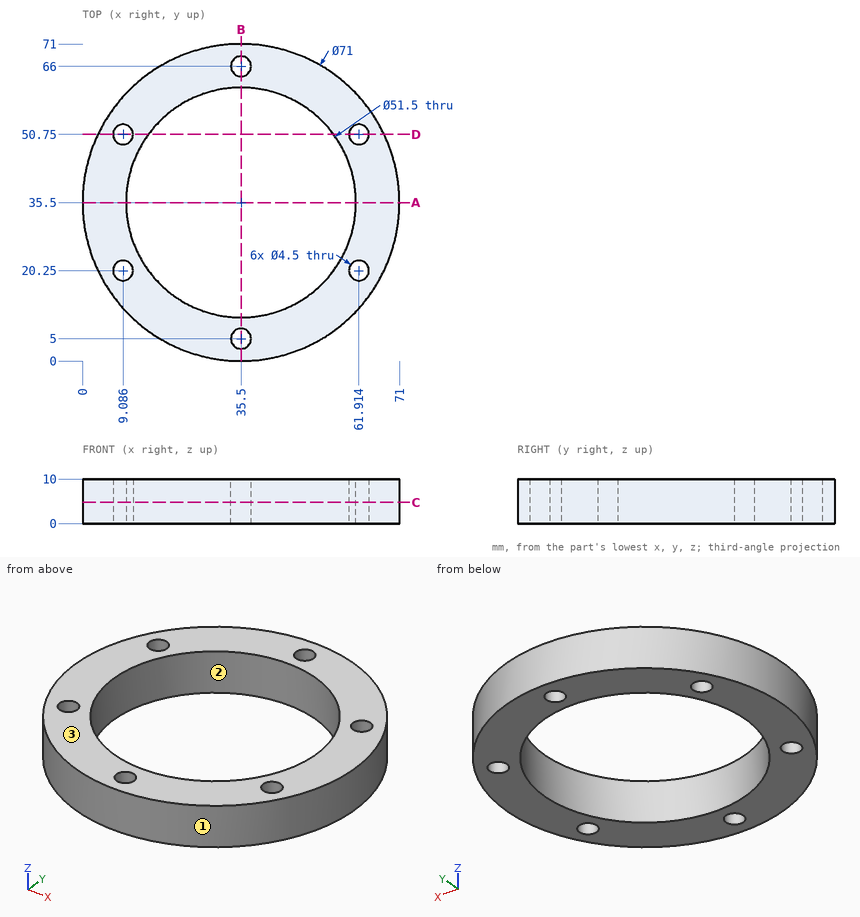
Study the drawing (mm; zero at the part's minimum x, y, z) and answer. Coordinates: 2 decimals unless noted, no trailing zeros. Write each loop counter-clockwise with the first axis right and the second up, starting at its lowest first coordinate (ties: lowest second). Pieces come first, ordered by that corner, then holes. Notation, with made-up numbers: M 51,2 L 84,2 A27 cw 84,41 Z; hole C 28,-39 d4. An arc over 180 degrees is marked long. Write each question's results on one line, items separated by ' | '.
Item 1: The part is cut by section C-C on z = 4.75. Determine the outline of the cut face in (x, y).
Answer below:
outline: C 35.5,35.5 d71; hole C 9.09,20.25 d4.5; hole C 9.09,50.75 d4.5; hole C 35.5,35.5 d51.5; hole C 35.5,5 d4.5; hole C 35.5,66 d4.5; hole C 61.91,20.25 d4.5; hole C 61.91,50.75 d4.5
Item 2: Given P1, Ø6, axis at x = 61.91, y = 20.25, coming from the -Z side; P2, Ø1.5, axis at x = 41.5, z = 4.5, coming from the -Y side; P3, Ø3, axis at x = 22.5, z = 7.5, coming from the -Y side; P4, Ø5, axis at x = 49.5, z = 2.5, coming from the +Y side, each flat-ended and moving along its own axis, determine where each tip first touches the part or whether it passes through.
Answer below:
P1: z = 0 | P2: y = 0.39 | P3: y = 1.91 | P4: y = 69.09
Item 3: The part is cut by section A-A on y = 35.5. Determine the outline of the cut face in (x, z), and give its area (3 significant figures).
Answer below:
outline: M 0,0 L 9.75,0 L 9.75,10 L 0,10 Z; M 61.25,0 L 71,0 L 71,10 L 61.25,10 Z | area: 195 mm2
Item 4: Consider probe 1 along X at (y, z) = (21, 3.5) (1 decimal); probe 2 along X at (y, z) = (9.5, 7.25); probe 3 along X at (y, z) = (13.5, 8.25). Determine where each line is inside the solid, lowest interval first. Write a range as [from, to].
Answer below:
probe 1: [3.1, 7], [11.2, 14.2], [56.8, 59.8], [64, 67.9] | probe 2: [11.33, 59.67] | probe 3: [7.64, 22.12], [48.88, 63.36]
Item 5: For a pull along Y with two mould halves and no side action, classify the marked faces 1, 2 and 3 as released by +Y, released by -Y, zero draft, split by the parting line, or undercut.
Answer below:
face 1: split by the parting line | face 2: undercut | face 3: zero draft
Item 6: The part is cut by section B-B on x = 35.5. Determine the outline of the cut face in (y, z), and give its area (3 significant figures).
Answer below:
outline: M 0,0 L 2.75,0 L 2.75,10 L 0,10 Z; M 7.25,0 L 9.75,0 L 9.75,10 L 7.25,10 Z; M 61.25,0 L 63.75,0 L 63.75,10 L 61.25,10 Z; M 68.25,0 L 71,0 L 71,10 L 68.25,10 Z | area: 105 mm2
Item 7: The part is cut by section D-D on y = 50.75. Determine the outline of the cut face in (x, z).
Answer below:
outline: M 3.44,0 L 6.84,0 L 6.84,10 L 3.44,10 Z; M 11.34,0 L 14.75,0 L 14.75,10 L 11.34,10 Z; M 56.25,0 L 59.66,0 L 59.66,10 L 56.25,10 Z; M 64.16,0 L 67.56,0 L 67.56,10 L 64.16,10 Z
